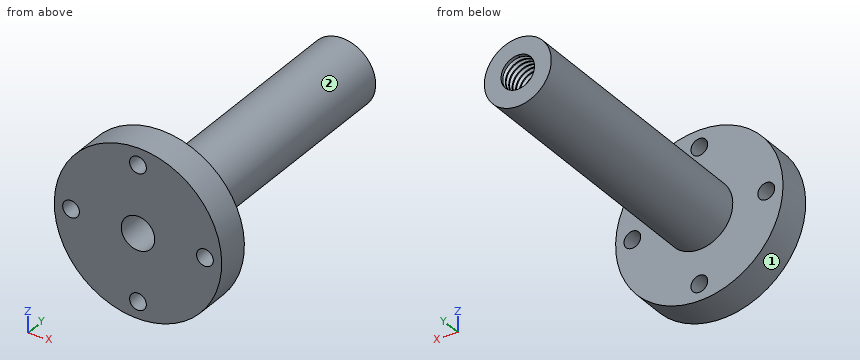
```python
from build123d import *

# Parameters (mm, degrees)
SKETCH1_R           = 25
BOSS_EXTRUDE1_DEPTH = 10
SKETCH2_R           = 10
BOSS_EXTRUDE2_DEPTH = 80
SKETCH3_R           = 5
CUT_EXTRUDE1_DEPTH  = 97.695398029
THREAD1_PITCH       = 1.5
THREAD1_HEIGHT      = 10
THREAD1_RADIUS      = 5
THREAD1_START_ANGLE = -90
SKETCH6_R           = 2.5
CUT_EXTRUDE2_DEPTH  = 97.695398122


with BuildPart() as part:
    # Sketch1 → Boss-Extrude1 (new body)
    with BuildSketch(Plane(origin=(0, 0, 0), x_dir=(1, 0, 0), z_dir=(0, 1, 0))):
        with Locations(Location((0, 0, 0), (0, 0, 270))):
            Circle(SKETCH1_R)
    extrude(amount=BOSS_EXTRUDE1_DEPTH)

    # Sketch2 → Boss-Extrude2 (add)
    with BuildSketch(Plane(origin=(0, 10, 0), x_dir=(1, 0, 0), z_dir=(0, 1, 0))):
        with Locations(Location((0, 0, 0), (0, 0, 270))):
            Circle(SKETCH2_R)
    extrude(amount=BOSS_EXTRUDE2_DEPTH)

    # Sketch3 → Cut-Extrude1 (cut, through all)
    with BuildSketch(Plane(origin=(0, 90, 0), x_dir=(1, 0, 0), z_dir=(0, 1, 0))):
        with Locations(Location((0, 0, 0), (0, 0, 270))):
            Circle(SKETCH3_R)
    extrude(amount=-CUT_EXTRUDE1_DEPTH, mode=Mode.SUBTRACT)

    # Thread1: sweep along a helix
    with BuildLine() as thread1_path:
        add(Helix(THREAD1_PITCH, THREAD1_HEIGHT, THREAD1_RADIUS, center=(0, 90, 0), direction=(0, -1, 0), mode=Mode.PRIVATE).rotate(Axis((0, 90, 0), (0, -1, 0)), THREAD1_START_ANGLE))
    # Thread Profile1 → Thread1 (sweep, cut)
    with BuildSketch(Plane(origin=(-5, 90, 0), x_dir=(-1, 0, 0), z_dir=(0, 0, 1))):
        Polygon((0, 0), (0.811898813, 0.468749998), (0.811898813, 0.656249998), (0, 1.124999996), align=None)
    sweep(path=thread1_path.line, is_frenet=True, mode=Mode.SUBTRACT)

    # Sketch6 → Cut-Extrude2 (cut, through all)
    with BuildSketch(Plane.XZ):
        with Locations(Location((0, 20, 0), (0, 0, 270))):
            Circle(SKETCH6_R)
        with Locations(Location((20, 0, 0), (0, 0, 270))):
            Circle(SKETCH6_R)
        with Locations(Location((0, -20, 0), (0, 0, 270))):
            Circle(SKETCH6_R)
        with Locations(Location((-20, 0, 0), (0, 0, 270))):
            Circle(SKETCH6_R)
    extrude(amount=-CUT_EXTRUDE2_DEPTH, mode=Mode.SUBTRACT)


solid = part.part
```
Can you work these out from the model? Positions are in its coordinate system, mm. Face numbers are marked on the shaded views. A direction names the side the tool comes from. Coordinates: 2 decimals unless noted, no trailing zeros. Loops run counter-clockwise (first coordinate to the right, second up) from the corner with the lowest first, then second, coordinate; pieces in that order, holes last. Notation, with made-up numbers: M 72.25,29 L 122.25,29 A24 ccw 122.25,63 Z; hole C 33,-25 d1. An arc over 180 degrees is marked long. Put each result on its own line as item: value. Start each with the question number.
(1) Will these pins go through, and if not, where does the flat tip stop? pin 1 Ø8 at (x, z) = (0, 20) entering from +Y; pin 2 Ø2 at (x, y) = (4, 45.5) entering from -Z; pin 3 Ø4 at (y, z) = (63, 7) entering from +X.
(2) Imagine slicing it at D-D on z = 7. List the corners of the cut face in (x, y) for me.
(3) Imagine slicing it at A-A on x = 20. List the corners of the cut face in (y, z) for me, and give its area (3 significant figures).
(4) Imagine slicing it at B-B on z = 20. List the corners of the cut face in (x, y) for me.
(5) I need wall thicknesses on probe 1 along X at (y, z) = (2, 0); probe 2 along X at (y, z) = (64, 0); probe 3 along Y at (x, z) = (-17, 4.5). Which ranges of each line are inside material? Lowest first, please.
(6) Imagine slicing it at C-C on y = 11. List the corners of the cut face in (x, z) for me, and give its area (3 significant figures).
(7) Which directions (+Z, -Z, +X, -X, +Y, -Y) give clear straight access to the entire face, cutting with the end or side of a thin tool? Please do the marked faces 1 and 2.
Worked answers:
1. pin 1: stops at y = 10
1. pin 2: stops at z = -9.54
1. pin 3: stops at x = 8.66
2. outline: M -24,0 L 24,0 L 24,10 L 7.14,10 L 7.14,90 L -7.14,90 L -7.14,10 L -24,10 Z
3. outline: M 0,-15 L 10,-15 L 10,-2.5 L 0,-2.5 Z; M 0,2.5 L 10,2.5 L 10,15 L 0,15 Z
3. area: 250 mm2
4. outline: M -15,0 L -2.5,0 L -2.5,10 L -15,10 Z; M 2.5,0 L 15,0 L 15,10 L 2.5,10 Z
5. probe 1: x = -25 to -22.5, -17.5 to -5, 5 to 17.5, 22.5 to 25
5. probe 2: x = -10 to -5, 5 to 10
5. probe 3: y = 0 to 10
6. outline: C 0,0 d20; hole C 0,0 d10
6. area: 236 mm2
7. face 1: +Y, -Y
7. face 2: +Y
